```python
from build123d import *

# Parameters (mm, degrees)
SKETCH1_W                                   = 100
SKETCH1_H                                   = 68
BOSS_EXTRUDE1_DEPTH                         = 6
SKETCH2_W                                   = 10
SKETCH2_H                                   = 25
CUT_EXTRUDE1_DEPTH                          = 61.761830124
SKETCH3_W                                   = 22
SKETCH3_H                                   = 14
CUT_EXTRUDE2_DEPTH                          = 61.761830124
SKETCH234_W                                 = 10
SKETCH234_H                                 = 6
BOSS_EXTRUDE234_DEPTH                       = 6
FILLET134_R                                 = 1
SKETCH2341_W                                = 10
SKETCH2341_H                                = 6
BOSS_EXTRUDE2341_DEPTH                      = 6
FILLET1341_R                                = 1
SKETCH2342_W                                = 10
SKETCH2342_H                                = 6
BOSS_EXTRUDE2342_DEPTH                      = 6
FILLET1342_R                                = 1
SKETCH6_W                                   = 10
SKETCH6_H                                   = 6
CUT_EXTRUDE11_DEPTH                         = 105.61109994
SKETCH62_W                                  = 10
SKETCH62_H                                  = 6
CUT_EXTRUDE13_DEPTH                         = 108.583694896
CUT_EXTRUDE110_START                        = -3
SKETCH67_W                                  = 6
SKETCH67_H                                  = 6
CUT_EXTRUDE110_DEPTH                        = 6
FILLET134_OF_MIRROR2_R                      = 1
FILLET1341_OF_MIRROR2_R                     = 1
FILLET1342_OF_MIRROR2_R                     = 1
SMART_FEATURE3_VIRTUAL_PIN_51_START         = 34
SMART_FEATURE3_VIRTUAL_PIN_51_OUTLINE_W     = 10
SMART_FEATURE3_VIRTUAL_PIN_51_OUTLINE_H     = 6
SMART_FEATURE3_VIRTUAL_PIN_51_DEPTH         = 6
SMART_FEATURE3_VIRTUAL_PIN_51_START_2       = 20
SMART_FEATURE3_VIRTUAL_PIN_51_2_OUTLINE_W   = 10
SMART_FEATURE3_VIRTUAL_PIN_51_2_OUTLINE_H   = 6
SMART_FEATURE3_VIRTUAL_PIN_51_2_OUTLINE_W_2 = 6
SMART_FEATURE3_VIRTUAL_PIN_51_2_DEPTH       = 6
CUT_EXTRUDE16_START                         = -3
CUT_EXTRUDE16_OUTLINE_W                     = 6
CUT_EXTRUDE16_OUTLINE_H                     = 10
CUT_EXTRUDE16_OUTLINE_H_2                   = 6
CUT_EXTRUDE16_OUTLINE_W_2                   = 10
CUT_EXTRUDE16_DEPTH                         = 6
CUT_EXTRUDE16_2_DEPTH                       = 6


# Read off the part's stored shape, not the designer's step: Smart-Feature3<virtual_pin-51>, Cut-Extrude16
with BuildPart() as part:
    # Sketch1 → Boss-Extrude1 (new body)
    with BuildSketch(Plane(origin=(0, 0, 0), x_dir=(1, 0, 0), z_dir=(0, 1, 0))):
        Rectangle(SKETCH1_W, SKETCH1_H)
    extrude(amount=BOSS_EXTRUDE1_DEPTH)

    # Sketch2 → Cut-Extrude1 (cut, through all)
    with BuildSketch(Plane.XZ):
        with Locations((16.4, -21.5)):
            Rectangle(SKETCH2_W, SKETCH2_H)
    cut_extrude1 = extrude(amount=-CUT_EXTRUDE1_DEPTH, mode=Mode.SUBTRACT)

    # Sketch3 → Cut-Extrude2 (cut, through all)
    with BuildSketch(Plane.XZ):
        with Locations((-14.6, -27)):
            Rectangle(SKETCH3_W, SKETCH3_H)
    cut_extrude2 = extrude(amount=-CUT_EXTRUDE2_DEPTH, mode=Mode.SUBTRACT)

    # Mirror1: Cut-Extrude1, Cut-Extrude2 across plane
    add(cut_extrude1.mirror(Plane.XY), mode=Mode.SUBTRACT)
    add(cut_extrude2.mirror(Plane.XY), mode=Mode.SUBTRACT)

    # Sketch234 → Boss-Extrude234 (add)
    with BuildSketch(Plane(origin=(34.932221392, 6, -34), x_dir=(1, 0, 0), z_dir=(0, 0, -1))):
        with Locations((0.767778608, 3)):
            Rectangle(SKETCH234_W, SKETCH234_H)
    boss_extrude234 = extrude(amount=BOSS_EXTRUDE234_DEPTH)

    # Fillet134
    fillet134_edges = [part.edges().sort_by_distance(p)[0] for p in [
        (40.7, 3, -40),
        (30.7, 3, -40),
    ]]
    fillet(fillet134_edges, radius=FILLET134_R)

    # Sketch2341 → Boss-Extrude2341 (add)
    with BuildSketch(Plane(origin=(3.132221392, 6, -34), x_dir=(1, 0, 0), z_dir=(0, 0, -1))):
        with Locations((0.767778608, 3)):
            Rectangle(SKETCH2341_W, SKETCH2341_H)
    boss_extrude2341 = extrude(amount=BOSS_EXTRUDE2341_DEPTH)

    # Fillet1341
    fillet1341_edges = [part.edges().sort_by_distance(p)[0] for p in [
        (8.9, 3, -40),
        (-1.1, 3, -40),
    ]]
    fillet(fillet1341_edges, radius=FILLET1341_R)

    # Sketch2342 → Boss-Extrude2342 (add)
    with BuildSketch(Plane(origin=(-38.567778608, 6, -34), x_dir=(1, 0, 0), z_dir=(0, 0, -1))):
        with Locations((0.767778608, 3)):
            Rectangle(SKETCH2342_W, SKETCH2342_H)
    boss_extrude2342 = extrude(amount=BOSS_EXTRUDE2342_DEPTH)

    # Fillet1342
    fillet1342_edges = [part.edges().sort_by_distance(p)[0] for p in [
        (-32.8, 3, -40),
        (-42.8, 3, -40),
    ]]
    fillet(fillet1342_edges, radius=FILLET1342_R)

    # Sketch6 → Cut-Extrude11 (cut, symmetric)
    with BuildSketch(Plane(origin=(34.932221392, 3, 21), x_dir=(1, 0, 0), z_dir=(0, -1, 0))):
        with Locations((0.767778608, -44)):
            Rectangle(SKETCH6_W, SKETCH6_H)
    cut_extrude11 = extrude(amount=CUT_EXTRUDE11_DEPTH, both=True, mode=Mode.SUBTRACT)

    # Sketch62 → Cut-Extrude13 (cut, symmetric)
    with BuildSketch(Plane(origin=(-38.567778608, 3, 21), x_dir=(1, 0, 0), z_dir=(0, -1, 0))):
        with Locations((0.767778608, -44)):
            Rectangle(SKETCH62_W, SKETCH62_H)
    cut_extrude13 = extrude(amount=CUT_EXTRUDE13_DEPTH, both=True, mode=Mode.SUBTRACT)

    # Sketch67 → Cut-Extrude110 (cut)
    with BuildSketch(Plane(origin=(3.132221392, 3, 21), x_dir=(1, 0, 0), z_dir=(0, -1, 0)).offset(CUT_EXTRUDE110_START)):
        with Locations((0.767778608, -44)):
            Rectangle(SKETCH67_W, SKETCH67_H)
    cut_extrude110 = extrude(amount=CUT_EXTRUDE110_DEPTH, mode=Mode.SUBTRACT)

    # Mirror2: Boss-Extrude234, Boss-Extrude2341, Boss-Extrude2342, Cut-Extrude11, Cut-Extrude13, Cut-Extrude110 across plane
    add(boss_extrude234.mirror(Plane.XY))
    add(boss_extrude2341.mirror(Plane.XY))
    add(boss_extrude2342.mirror(Plane.XY))
    add(cut_extrude11.mirror(Plane.XY), mode=Mode.SUBTRACT)
    add(cut_extrude13.mirror(Plane.XY), mode=Mode.SUBTRACT)
    add(cut_extrude110.mirror(Plane.XY), mode=Mode.SUBTRACT)

    # Fillet134 of Mirror2
    fillet134_of_mirror2_edges = [part.edges().sort_by_distance(p)[0] for p in [
        (40.7, 3, 40),
        (30.7, 3, 40),
    ]]
    fillet(fillet134_of_mirror2_edges, radius=FILLET134_OF_MIRROR2_R)

    # Fillet1341 of Mirror2
    fillet1341_of_mirror2_edges = [part.edges().sort_by_distance(p)[0] for p in [
        (8.9, 3, 40),
        (-1.1, 3, 40),
    ]]
    fillet(fillet1341_of_mirror2_edges, radius=FILLET1341_OF_MIRROR2_R)

    # Fillet1342 of Mirror2
    fillet1342_of_mirror2_edges = [part.edges().sort_by_distance(p)[0] for p in [
        (-32.8, 3, 40),
        (-42.8, 3, 40),
    ]]
    fillet(fillet1342_of_mirror2_edges, radius=FILLET1342_OF_MIRROR2_R)

    # Smart-Feature3<virtual_pin-51> outline → Smart-Feature3<virtual_pin-51> (cut)
    with BuildSketch(Plane.XY.offset(SMART_FEATURE3_VIRTUAL_PIN_51_START)):
        with Locations((35.7, 3)):
            Rectangle(SMART_FEATURE3_VIRTUAL_PIN_51_OUTLINE_W, SMART_FEATURE3_VIRTUAL_PIN_51_OUTLINE_H)
        with Locations((3.9, 3)):
            Rectangle(SMART_FEATURE3_VIRTUAL_PIN_51_OUTLINE_W, SMART_FEATURE3_VIRTUAL_PIN_51_OUTLINE_H)
        with Locations((-37.8, 3)):
            Rectangle(SMART_FEATURE3_VIRTUAL_PIN_51_OUTLINE_W, SMART_FEATURE3_VIRTUAL_PIN_51_OUTLINE_H)
    extrude(amount=SMART_FEATURE3_VIRTUAL_PIN_51_DEPTH, mode=Mode.SUBTRACT)

    # Smart-Feature3_virtual_pin-51 2 outline → Smart-Feature3_virtual_pin-51 2 (add)
    with BuildSketch(Plane.XY.offset(SMART_FEATURE3_VIRTUAL_PIN_51_START_2)):
        with Locations((35.7, 3)):
            Rectangle(SMART_FEATURE3_VIRTUAL_PIN_51_2_OUTLINE_W, SMART_FEATURE3_VIRTUAL_PIN_51_2_OUTLINE_H)
        with Locations((3.9, 3)):
            Rectangle(SMART_FEATURE3_VIRTUAL_PIN_51_2_OUTLINE_W_2, SMART_FEATURE3_VIRTUAL_PIN_51_2_OUTLINE_H)
        with Locations((-37.8, 3)):
            Rectangle(SMART_FEATURE3_VIRTUAL_PIN_51_2_OUTLINE_W, SMART_FEATURE3_VIRTUAL_PIN_51_2_OUTLINE_H)
    extrude(amount=SMART_FEATURE3_VIRTUAL_PIN_51_2_DEPTH)

    # Cut-Extrude16 outline → Cut-Extrude16 (cut)
    with BuildSketch(Plane(origin=(-76, 3, -3.232221392), x_dir=(0, 0, -1), z_dir=(0, 1, 0)).offset(CUT_EXTRUDE16_START)):
        with Locations((-26.232221392, -111.7)):
            Rectangle(CUT_EXTRUDE16_OUTLINE_W, CUT_EXTRUDE16_OUTLINE_H)
        with Locations((-26.232221392, -38.2)):
            Rectangle(CUT_EXTRUDE16_OUTLINE_W, CUT_EXTRUDE16_OUTLINE_H)
        with Locations((-26.232221392, -79.9)):
            Rectangle(CUT_EXTRUDE16_OUTLINE_W, CUT_EXTRUDE16_OUTLINE_H_2)
        with Locations((0.767778608, -44)):
            Rectangle(CUT_EXTRUDE16_OUTLINE_W_2, CUT_EXTRUDE16_OUTLINE_H_2)
    extrude(amount=CUT_EXTRUDE16_DEPTH, mode=Mode.SUBTRACT)

    # Cut-Extrude16 2 outline → Cut-Extrude16 2 (add)
    with BuildSketch(Plane(origin=(-76, 3, -3.232221392), x_dir=(0, 0, -1), z_dir=(0, 1, 0)).offset(CUT_EXTRUDE16_START)):
        with BuildLine():
            ThreePointArc((-43.232221392, -115.7), (-42.939328173, -116.407106781), (-42.232221392, -116.7))
            Line((-42.232221392, -116.7), (-37.232221392, -116.7))
            Line((-37.232221392, -116.7), (-37.232221392, -106.7))
            Line((-37.232221392, -106.7), (-42.232221392, -106.7))
            ThreePointArc((-42.232221392, -106.7), (-42.939328173, -106.992893219), (-43.232221392, -107.7))
            Line((-43.232221392, -107.7), (-43.232221392, -115.7))
        make_face()
        with BuildLine():
            ThreePointArc((-43.232221392, -83.9), (-42.939328173, -84.607106781), (-42.232221392, -84.9))
            Line((-42.232221392, -84.9), (-37.232221392, -84.9))
            Line((-37.232221392, -84.9), (-37.232221392, -74.9))
            Line((-37.232221392, -74.9), (-42.232221392, -74.9))
            ThreePointArc((-42.232221392, -74.9), (-42.939328173, -75.192893219), (-43.232221392, -75.9))
            Line((-43.232221392, -75.9), (-43.232221392, -83.9))
        make_face()
        with BuildLine():
            ThreePointArc((-43.232221392, -42.2), (-42.939328173, -42.907106781), (-42.232221392, -43.2))
            Line((-42.232221392, -43.2), (-37.232221392, -43.2))
            Line((-37.232221392, -43.2), (-37.232221392, -33.2))
            Line((-37.232221392, -33.2), (-42.232221392, -33.2))
            ThreePointArc((-42.232221392, -33.2), (-42.939328173, -33.492893219), (-43.232221392, -34.2))
            Line((-43.232221392, -34.2), (-43.232221392, -42.2))
        make_face()
    extrude(amount=CUT_EXTRUDE16_2_DEPTH)


solid = part.part
```
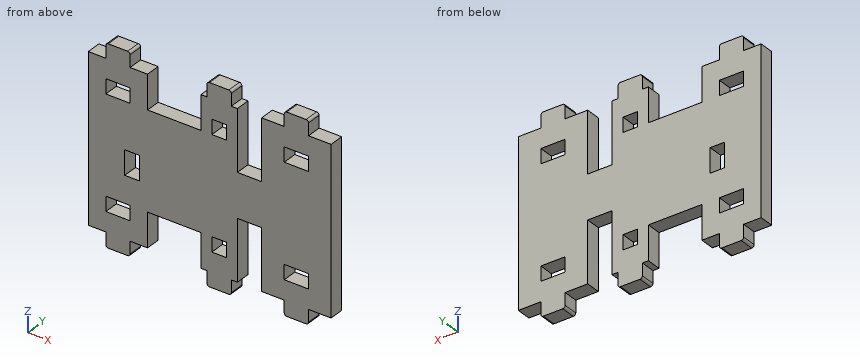
Here's how the part is built. I have some questions about the finished solid (model axes, mm). Coordinates: 2 decimals unless noted, no trailing zeros. Loops run counter-clockwise (first coordinate to the right, second up) from the corner with the lowest first, then second, coordinate; pieces in that order, holes last. Notation, with made-up numbers: (53.25, 27) - (62.25, 27) arc R15 ccw to (62.25, 39) - close; hole circle Ø4 at (54, 28). An arc over 180 degrees is marked (long way). Return JSON: item names as keys, results as strings. Group by question number.
Item 1: I need wall thicknesses on line 1 (Z direction, x = -38, y = 3.35); line 2 (X direction, y = 5.7, z = 25.5); line 3 (X direction, y = 1.3, z = -27). Which ranges of each line are inside material? Lowest first, please. Write a range as from..to.
Item 2: If we section it at B-B on z = 30: Write out the boundary of the cut face in (x, y).
Item 3: Will these pins go through, and if not, where does the flat tip stop? P1, Ø1, axis at x = 37.5, z = 8.5, coming from the -Y side; P2, Ø1.8, axis at x = -30, y = 2.5, coming from the +Z side; P3, Ø1.5, axis at y = 3, z = -37, coming from the +X side; P4, Ø3, axis at x = -18, y = 5, coming from the +Z side.
Item 4: If we section it at D-D on y = 3.6: State how many separate pieces and enclosed holes the cut face has, and give its area (3 significant figures).
Item 5: If we section it at A-A on z = -16: Write out the boundary of the cut face in (x, y).
Item 6: If we section it at C-C on x = 36: Write out the boundary of the cut face in (y, z).
Calculated:
{
 "1": {"line 1": "z = -40..-26, -20..20, 26..40", "line 2": "x = -50..-42.8, -32.8..-25.6, -3.6..0.9, 6.9..11.4, 21.4..30.7, 40.7..50", "line 3": "x = -50..-25.6, -3.6..11.4, 21.4..50"},
 "2": {"outline": "(-50, 0) - (-25.6, 0) - (-25.6, 6) - (-50, 6) - close; (-3.6, 0) - (11.4, 0) - (11.4, 6) - (-3.6, 6) - close; (21.4, 0) - (50, 0) - (50, 6) - (21.4, 6) - close"},
 "3": {"P1": "stops at y = 0", "P2": "stops at z = 34", "P3": "stops at x = 40.7", "P4": "stops at z = 20"},
 "4": {"separate pieces": "1", "enclosed holes": "7", "area": "5,670 mm^2"},
 "5": {"outline": "(-50, 0) - (11.4, 0) - (11.4, 6) - (-50, 6) - close; (21.4, 0) - (50, 0) - (50, 6) - (21.4, 6) - close"},
 "6": {"outline": "(0, -40) - (6, -40) - (6, -26) - (0, -26) - close; (0, -20) - (6, -20) - (6, 20) - (0, 20) - close; (0, 26) - (6, 26) - (6, 40) - (0, 40) - close"}
}
